from build123d import *

# Parameters (mm, degrees)
SKETCH1_R           = 1.5875
SKETCH1_W           = 3.302
SKETCH1_H           = 7.747
BOSS_EXTRUDE1_DEPTH = 3.175
SKETCH3_W           = 3.175
SKETCH3_H           = 2.54
CUT_EXTRUDE1_DEPTH  = 3.175
FILLET1_R           = 6.35
FILLET2_R           = 6.35
FILLET3_R           = 6.35


with BuildPart() as part:
    # Sketch1 → Boss-Extrude1 (new body)
    with BuildSketch(Plane(origin=(0, 0, 0), x_dir=(1, 0, 0), z_dir=(0, 1, 0))):
        Polygon((30.48, 6.35), (-17.78, 6.35), (-17.78, 25.4), (-30.48, 25.4), (-30.48, 6.35), (-30.48, -6.35), (30.48, -6.35), align=None)
        with Locations(Location((-24.13, 22.225, 0), (0, 0, 270))):
            Circle(SKETCH1_R, mode=Mode.SUBTRACT)
        with Locations((-9.906, 0)):
            Rectangle(SKETCH1_W, SKETCH1_H, mode=Mode.SUBTRACT)
    extrude(amount=BOSS_EXTRUDE1_DEPTH)

    # Sketch3 → Cut-Extrude1 (cut)
    with BuildSketch(Plane(origin=(0, 3.175, 0), x_dir=(1, 0, 0), z_dir=(0, 1, 0))):
        with Locations((28.8925, 5.08)):
            Rectangle(SKETCH3_W, SKETCH3_H)
        with Locations((28.8925, -5.08)):
            Rectangle(SKETCH3_W, SKETCH3_H)
    extrude(amount=-CUT_EXTRUDE1_DEPTH, mode=Mode.SUBTRACT)

    # Fillet1
    fillet1_edges = [part.edges().sort_by_distance(p)[0] for p in [
        (-30.48, 1.5875, -25.4),
    ]]
    fillet(fillet1_edges, radius=FILLET1_R)

    # Fillet2
    fillet2_edges = [part.edges().sort_by_distance(p)[0] for p in [
        (-17.78, 1.5875, -25.4),
    ]]
    fillet(fillet2_edges, radius=FILLET2_R - 0.0001)  # a hair under: the kernel refuses the full size

    # Fillet3
    fillet3_edges = [part.edges().sort_by_distance(p)[0] for p in [
        (-30.48, 1.5875, 6.35),
    ]]
    fillet(fillet3_edges, radius=FILLET3_R)


solid = part.part
Check sheet for the modelled part. Datum: model origin and axes. Units: mm. A direction names the side the tool comes from. Round coordinates to 2 decimals unless told otherwise and drop trailing zeros. Loops run counter-clockwise (first coordinate to the right, second up) from the corner with the lowest first, then second, coordinate; pieces in that order, holes last. Notation, with made-up numbers: M -11,65 L -5,65 A25 cw -5,87 Z; hole C 60.5,46.25 d6. An arc over 180 degrees is marked long. One line per item, written item: value.
(1) Thickness scan on line 1 (X direction, y = 1.85, z = -2) (3 decimals); line 2 (Z direction, x = 0, y = 2.1); line 3 (X direction, y = 0.65, z = -16). Record the ranges inside material, lowest first.
Computed values:
line 1: x = -30.48 to -11.557, -8.255 to 30.48
line 2: z = -6.35 to 6.35
line 3: x = -30.48 to -17.78
(2) Release check for a two-part mould opening along X. For faces 1 (the face through (-10, 2, 3.874)), 2 (the face through (27.305, 2, -5)), 3 (the face through (-8.255, 2, 0)), 4 (the face through (29, 2, 3.81)) record: +X half, -X half, draft (parallel to the pull), parting line (faces both ways), or undercut.
Computed values:
face 1: undercut
face 2: +X half
face 3: undercut
face 4: draft
(3) Sectioned sample at C-C, the plane z = 1. Record the cut outline in (x, y) (3 decimals), then the cut area to 3 significant figures.
Computed values:
outline: M -30.401,0 L -11.557,0 L -11.557,3.175 L -30.401,3.175 Z; M -8.255,0 L 30.48,0 L 30.48,3.175 L -8.255,3.175 Z
area: 183 mm^2
(4) Depth check by flat-ended pin: pin 1 Ø1.5 at (y, z) = (2.5, -20) entering from -X; pin 2 Ø0.8 at (y, z) = (1, 5) entering from +X (3 decimals); pin 3 Ø1 at (x, y) = (29.5, 2) entering from +Z. Enter the tip coordinate at first touch or a pass-through.
Computed values:
pin 1: stops at x = -30.48
pin 2: stops at x = 27.305
pin 3: stops at z = 3.81
(5) Sectioned sample at B-B, the plane z = -2.5. Record the cut outline in (x, y) (3 decimals), then the cut area to 3 significant figures.
Computed values:
outline: M -30.48,0 L -11.557,0 L -11.557,3.175 L -30.48,3.175 Z; M -8.255,0 L 30.48,0 L 30.48,3.175 L -8.255,3.175 Z
area: 183 mm^2
(6) Access from +Z, -Z, +X, -X, +Y, -Y to the whole of each face (thin tool, end or side, straight path). Record for faces 5 (the face through (-17.78, 2, -13)), 6 (the face through (27.305, 2, 5)), 7 (the face through (-10, 2, -3.874)).
Computed values:
face 5: -Z, +X, +Y, -Y
face 6: +Z, +X, +Y, -Y
face 7: +Y, -Y
(7) Sectioned sample at D-D, the plane x = 15.5. Record the cut outline in (y, z) (3 decimals), then the cut area to 3 significant figures.
Computed values:
outline: M 0,-6.35 L 3.175,-6.35 L 3.175,6.35 L 0,6.35 Z
area: 40.3 mm^2
(8) Sectioned sample at A-A, the plane y = 1.35. Count the separate pieces of the cut face and the enclosed holes in it, then the cut area to 3 significant figures.
Computed values:
separate pieces: 1
enclosed holes: 2
area: 941 mm^2
